Check sheet for the modelled part. Datum: model origin and axes. Units: mm. A direction names the side the tool comes from. Coordinates: 2 decimals unless noted, no trailing zeros. Order: outer loops, then holes, each group sorted by start corner. A loop starts at its lowest first (then second) coordinate and runs counter-clockwise, first axis right, second up.
from build123d import *

# Parameters (mm, degrees)
SKETCH10_W                                           = 31.75
SKETCH10_H                                           = 31.75
SKETCH10_W_2                                         = 2.54
SKETCH10_H_2                                         = 5.08
SKETCH10_W_3                                         = 5.08
SKETCH10_H_3                                         = 2.54
BOSS_EXTRUDE3_DEPTH                                  = 12.7
SKETCH11_W                                           = 31.75
SKETCH11_H                                           = 31.75
BOSS_EXTRUDE4_DEPTH                                  = 76.2
CBORE_FOR_1_4_BINDING_HEAD_MACHINE_SCREW_D           = 6.7564
CBORE_FOR_1_4_BINDING_HEAD_MACHINE_SCREW_CBORE_D     = 14.2875
CBORE_FOR_1_4_BINDING_HEAD_MACHINE_SCREW_CBORE_DEPTH = 69.85
CUT_EXTRUDE1_DEPTH                                   = 31.75


with BuildPart() as part:
    # Sketch10 → Boss-Extrude3 (new body)
    # profile 1 of 9: a face of its own
    with BuildSketch(Plane(origin=(0, 0, 0), x_dir=(0, 0, -1), z_dir=(1, 0, 0))):
        Rectangle(SKETCH10_W, SKETCH10_H)
        Polygon((-2.54, 12.7), (2.54, 12.7), (12.7, 12.7), (12.7, 2.54), (12.7, -2.54), (12.7, -12.7), (2.54, -12.7), (-2.54, -12.7), (-12.7, -12.7), (-12.7, -2.54), (-12.7, 2.54), (-12.7, 12.7), align=None, mode=Mode.SUBTRACT)
    # profile 2 of 9: a face of its own
    with BuildSketch(Plane(origin=(0, 0, 0), x_dir=(0, 0, -1), z_dir=(1, 0, 0))):
        with Locations((11.43, 0)):
            Rectangle(SKETCH10_W_2, SKETCH10_H_2)
    # profile 3 of 9: a face of its own
    with BuildSketch(Plane(origin=(0, 0, 0), x_dir=(0, 0, -1), z_dir=(1, 0, 0))):
        with BuildLine():
            Line((10.16, -2.54), (10.16, 2.54))
            Line((10.16, 2.54), (10.16, 6.35))
            ThreePointArc((10.16, 6.35), (10.012022021, 6.580814495), (9.740509205, 6.542688341))
            Line((9.740509205, 6.542688341), (5.08, 2.54))
            Line((5.08, 2.54), (5.08, -2.54))
            Line((5.08, -2.54), (9.740509205, -6.542688341))
            ThreePointArc((9.740509205, -6.542688341), (10.012022021, -6.580814495), (10.16, -6.35))
            Line((10.16, -6.35), (10.16, -2.54))
        make_face()
    # profile 4 of 9: a face of its own
    with BuildSketch(Plane(origin=(0, 0, 0), x_dir=(0, 0, -1), z_dir=(1, 0, 0))):
        with Locations((0, -11.43)):
            Rectangle(SKETCH10_W_3, SKETCH10_H_3)
    # profile 5 of 9: a face of its own
    with BuildSketch(Plane(origin=(0, 0, 0), x_dir=(0, 0, -1), z_dir=(1, 0, 0))):
        with BuildLine():
            ThreePointArc((6.542688341, -9.740509205), (6.580814495, -10.012022021), (6.35, -10.16))
            Line((6.35, -10.16), (-6.35, -10.16))
            ThreePointArc((-6.35, -10.16), (-6.580814495, -10.012022021), (-6.542688341, -9.740509205))
            Line((-6.542688341, -9.740509205), (-2.54, -5.08))
            Line((-2.54, -5.08), (2.54, -5.08))
            Line((2.54, -5.08), (6.542688341, -9.740509205))
        make_face()
    # profile 6 of 9: a face of its own
    with BuildSketch(Plane(origin=(0, 0, 0), x_dir=(0, 0, -1), z_dir=(1, 0, 0))):
        with Locations((0, 11.43)):
            Rectangle(SKETCH10_W_3, SKETCH10_H_3)
    # profile 7 of 9: a face of its own
    with BuildSketch(Plane(origin=(0, 0, 0), x_dir=(0, 0, -1), z_dir=(1, 0, 0))):
        with BuildLine():
            Line((6.35, 10.16), (-6.35, 10.16))
            ThreePointArc((-6.35, 10.16), (-6.580814495, 10.012022021), (-6.542688341, 9.740509205))
            Line((-6.542688341, 9.740509205), (-2.54, 5.08))
            Line((-2.54, 5.08), (2.54, 5.08))
            Line((2.54, 5.08), (6.542688341, 9.740509205))
            ThreePointArc((6.542688341, 9.740509205), (6.580814495, 10.012022021), (6.35, 10.16))
        make_face()
    # profile 8 of 9: a face of its own
    with BuildSketch(Plane(origin=(0, 0, 0), x_dir=(0, 0, -1), z_dir=(1, 0, 0))):
        with BuildLine():
            Line((-5.08, 2.54), (-9.740509205, 6.542688341))
            ThreePointArc((-9.740509205, 6.542688341), (-10.012022021, 6.580814495), (-10.16, 6.35))
            Line((-10.16, 6.35), (-10.16, -6.35))
            ThreePointArc((-10.16, -6.35), (-10.012022021, -6.580814495), (-9.740509205, -6.542688341))
            Line((-9.740509205, -6.542688341), (-5.08, -2.54))
            Line((-5.08, -2.54), (-5.08, 2.54))
        make_face()
    # profile 9 of 9: a face of its own
    with BuildSketch(Plane(origin=(0, 0, 0), x_dir=(0, 0, -1), z_dir=(1, 0, 0))):
        with Locations((-11.43, 0)):
            Rectangle(SKETCH10_W_2, SKETCH10_H_2)
    extrude(amount=-BOSS_EXTRUDE3_DEPTH)

    # Sketch11 → Boss-Extrude4 (add)
    with BuildSketch(Plane(origin=(0, 0, 0), x_dir=(0, 0, -1), z_dir=(1, 0, 0))):
        Rectangle(SKETCH11_W, SKETCH11_H)
    extrude(amount=BOSS_EXTRUDE4_DEPTH)

    # CBORE for 1/4 Binding Head Machine Screw1 (through all)
    with Locations(Plane(origin=(76.2, 0, 0), x_dir=(0, 0, -1), z_dir=(1, 0, 0))):
        with Locations((0, 0)):
            CounterBoreHole(CBORE_FOR_1_4_BINDING_HEAD_MACHINE_SCREW_D / 2, CBORE_FOR_1_4_BINDING_HEAD_MACHINE_SCREW_CBORE_D / 2, CBORE_FOR_1_4_BINDING_HEAD_MACHINE_SCREW_CBORE_DEPTH)

    # Sketch15 → Cut-Extrude1 (cut)
    with BuildSketch(Plane(origin=(0, 15.875, 0), x_dir=(1, 0, 0), z_dir=(0, 1, 0))):
        with BuildLine():
            Line((76.2, 15.875), (76.2, -15.875))
            ThreePointArc((76.2, -15.875), (60.325, 0), (76.2, 15.875))
        make_face()
    extrude(amount=-CUT_EXTRUDE1_DEPTH, mode=Mode.SUBTRACT)


solid = part.part
(1) Cross-section at B-B (z = 0). Enter the section's corners in (x, y) (3 decimals).
Filled in:
outline: (-12.7, -15.875) - (60.325, -15.875) - (60.325, -7.144) - (6.35, -7.144) - (6.35, -3.378) - (0, -3.378) - (0, -5.08) - (-12.7, -5.08) - close; (-12.7, 5.08) - (0, 5.08) - (0, 3.378) - (6.35, 3.378) - (6.35, 7.144) - (60.325, 7.144) - (60.325, 15.875) - (-12.7, 15.875) - close
(2) Cross-section at A-A (y = 0). Enter the section's corners in (x, z) (3 decimals).
Filled in:
outline: (-12.7, -15.875) - (76.2, -15.875) arc R15.875 cw to (62.023, -7.144) - (6.35, -7.144) - (6.35, -3.378) - (0, -3.378) - (0, -5.08) - (-12.7, -5.08) - close; (-12.7, 5.08) - (0, 5.08) - (0, 3.378) - (6.35, 3.378) - (6.35, 7.144) - (62.023, 7.144) arc R15.875 cw to (76.2, 15.875) - (-12.7, 15.875) - close
(3) Thickness scan on probe 1 along Y at (x, z) = (28.5, 0) (3 decimals); probe 2 along Y at (x, z) = (3, 0) (3 decimals). Record the ranges inside material, lowest first.
Filled in:
probe 1: y = -15.875 to -7.144, 7.144 to 15.875
probe 2: y = -15.875 to -3.378, 3.378 to 15.875
(4) Release check for a two-part mould opening along Y. For faces 3 (the flat face through (21, 15.875, 0)), 4 (the flat face through (31, 0, 15.875)), 5 (the flat face through (-6, 4, -10.16)) record: +Y half, -Y half, draft (parallel to the pull), parting line (faces both ways), or undercut.
Filled in:
face 3: +Y half
face 4: draft
face 5: undercut
(5) Cross-section at D-D (x = 64). Enter the section's corners in (y, z) (3 decimals), and give its area (3 significant figures).
Filled in:
outline: (-15.875, -15.875) - (15.875, -15.875) - (15.875, -10.158) - (-15.875, -10.158) - close; (-15.875, 10.158) - (15.875, 10.158) - (15.875, 15.875) - (-15.875, 15.875) - close
area: 363 mm2
(6) Cross-section at C-C (x = 8.5). Enter the section's corners in (y, z) (1 decimal), and give its area (3 significant figures).
Filled in:
outline: (-15.9, -15.9) - (15.9, -15.9) - (15.9, 15.9) - (-15.9, 15.9) - close; hole circle Ø14.3 at (0, 0)
area: 848 mm2
(7) Tool access check on faces 1 (the flat face through (31, 0, -15.875)), 2 (the flat face through (-6, 12.7, 8)). Record the directions out of +Z, -Z, +X, -X, +Y, -Y that give a thin tool (end or side, any length) a straight path to the whole face; none if there is none.
Filled in:
face 1: -Z, +X, -X, +Y, -Y
face 2: -X
(8) Go/stop test with flat-tipped pins: P1, Ø8.5, axis at y = 0, z = 0, coming from the -X side; P2, Ø6, axis at y = -1.5, z = -2, coming from the +X side; P3, Ø11.5, axis at y = 1, z = 1.5, coming from the +X side. Record where each tip stops, or that it passes through.
Filled in:
P1: stops at x = 0
P2: stops at x = 6.35
P3: stops at x = 62.08
